For this review, use the dimensioned drawing (mm, ordinates from the lowest corner) and the shaded views. A direction names the side the tool comes from. Coordinates: 2 decimals unless noted, no trailing zeros. Loops run counter-clockwise (first coordinate to the right, second up) from the corner with the lowest first, then second, coordinate; pieces in that order, holes last. Notation, with made-up numbers: M -19,68 L 31,68 A11 cw 31,83 Z; hole C -40,40 d8. An arc over 180 degrees is marked long. Write item = value, one per line.
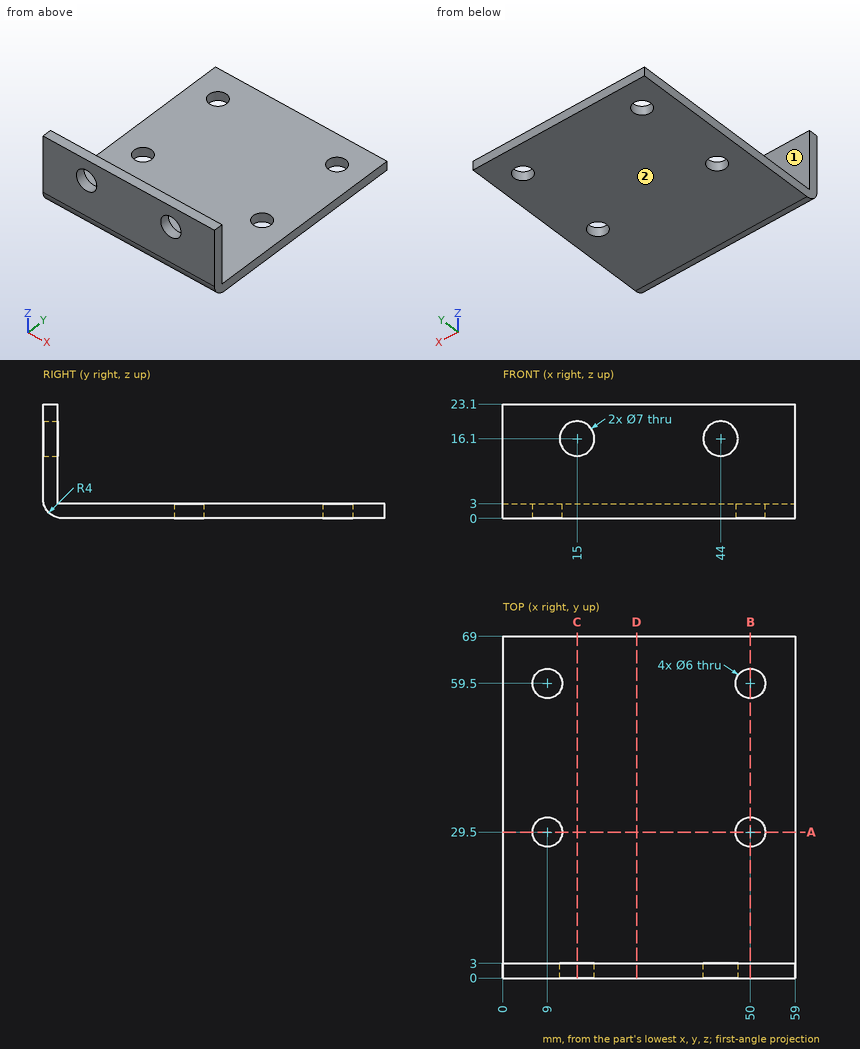
Q1. For pin 1 Ø8 at (y, z) = (53, 7.5) entering from -X; pin 2 Ø8 at (x, z) = (9, 20) entering from +Y; pin 3 Ø1.5 at (x, y) = (37.5, 38.5) entering from +Z; pin 4 Ø8 at (x, z) = (15, 16.1) entering from -Y, all flat-tipped, find the tip position at first contact; note any pin that passes through.
Solved:
pin_1 = through
pin_2 = 3
pin_3 = 3
pin_4 = 0
Q2. Add section A-A (y = 29.5). Write out the cut boundary in (x, z), and give its area (3 significant figures).
Solved:
outline = M 0,0 L 6,0 L 6,3 L 0,3 Z; M 12,0 L 47,0 L 47,3 L 12,3 Z; M 53,0 L 59,0 L 59,3 L 53,3 Z
area = 141 mm²
Q3. Add section B-B (x = 50). Write out the cut boundary in (y, z), and give its area (3 significant figures).
Solved:
outline = M 0,4 A4 ccw 4,0 L 26.5,0 L 26.5,3 L 3,3 L 3,23.1 L 0,23.1 Z; M 32.5,0 L 56.5,0 L 56.5,3 L 32.5,3 Z; M 62.5,0 L 69,0 L 69,3 L 62.5,3 Z
area = 228 mm²
Q4. Add section D-D (x = 27). Write out the cut boundary in (y, z), and give its area (3 significant figures).
Solved:
outline = M 0,4 A4 ccw 4,0 L 69,0 L 69,3 L 3,3 L 3,23.1 L 0,23.1 Z
area = 264 mm²
Q5. Add section C-C (x = 15). Write out the cut boundary in (y, z), and give its area (3 significant figures).
Solved:
outline = M 0,4 A4 ccw 4,0 L 69,0 L 69,3 L 3,3 L 3,12.6 L 0,12.6 Z; M 0,19.6 L 3,19.6 L 3,23.1 L 0,23.1 Z
area = 243 mm²
Q6. For line 1 along X through (y, z) = (29.5, 1.75); line 2 along Y through (x, z) = (50, 2.3); line 3 along Y through (x, z) = (9, 1.65), list the stretches that pass through material, from the lowest coordinate up.
Solved:
line_1 = 0 to 6, 12 to 47, 53 to 59
line_2 = 0.38 to 26.5, 32.5 to 56.5, 62.5 to 69
line_3 = 0.76 to 26.5, 32.5 to 56.5, 62.5 to 69
Q7. Machinability: for the marked faces 1 and 2, which of the approach directions +Z, -Z, +X, -X, +Y, -Y give a long, thin tool a straight path to every point of the face, cutting with its end or side? Answer none if there is none.
Solved:
face_1 = +Z, +X, -X, +Y
face_2 = -Z, +X, -X, +Y, -Y
